```python
from build123d import *

# Parameters (mm, degrees)
BOSS_EXTRUDE1_DEPTH = 44
SHELL1_T            = -2
CUT_EXTRUDE1_DEPTH  = 1


with BuildPart() as part:
    # Sketch1 → Boss-Extrude1 (new body)
    with BuildSketch(Plane(origin=(0, 0, 0), x_dir=(1, 0, 0), z_dir=(0, 1, 0))):
        with BuildLine():
            Line((0, -50), (0, -150))
            ThreePointArc((0, -150), (-86.602540378, -122.474487139), (-141.421356237, -50))
            Line((-141.421356237, -50), (0, -50))
        make_face()
    extrude(amount=BOSS_EXTRUDE1_DEPTH)

    # Shell1
    shell1_openings = [part.faces().sort_by_distance(p)[0] for p in [
        (-56.564232989, 0, 91.421606215),
        (-70.710678119, 22, 50),
        (0, 22, 100),
    ]]
    offset(amount=SHELL1_T, openings=shell1_openings, kind=Kind.INTERSECTION)

    # Sketch3 → Cut-Extrude1 (cut)
    with BuildSketch(Plane.XZ.offset(-42)):
        with BuildLine():
            Line((-139.298241195, 50), (0, 50))
            Line((0, 50), (0, 70))
            Line((0, 70), (-130.399386502, 70))
            ThreePointArc((-130.399386502, 70), (-135.219091094, 60.16475217), (-139.298241195, 50))
        make_face()
    extrude(amount=-CUT_EXTRUDE1_DEPTH, mode=Mode.SUBTRACT)


solid = part.part
```
The model under review builds one solid part; all positions refer to its coordinate system, in mm. A direction names the side the tool comes from. Round coordinates to 2 decimals unless told otherwise and drop trailing zeros. Loops run counter-clockwise (first coordinate to the right, second up) from the corner with the lowest first, then second, coordinate; pieces in that order, holes last. Notation, with made-up numbers: M 73.5,13.25 L 109.5,13.25 A15 ccw 109.5,23.25 Z; hole C 6,37.5 d1. An arc over 180 degrees is marked long. Write item = value, one per line.
Item 1: Take a section at C-C on y = 20. Write out the cut boundary in (x, z), then the cut area to 3 significant figures.
Return value:
outline = M -141.42,50 L -139.3,50 A148 cw 0,148 L 0,150 A150 ccw Z
area = 366 mm2
Item 2: Take a section at B-B on z = 119.5. Write out the cut boundary in (x, y).
Return value:
outline = M -90.66,0 L -87.31,0 L -87.31,42 L 0,42 L 0,44 L -90.66,44 Z
Item 3: Machinability: for faces 1 (the cylindrical face through (-85.54, 21.69, 123.22)), 2 (the flat face through (-71, 43, 60)), which of the approach directions +Z, -Z, +X, -X, +Y, -Y give a long, thin tool a straight path to every point of the face, cutting with its end or side? Answer none if there is none.
Return value:
face_1 = +Z, -X, +Y, -Y
face_2 = -Z, +X, -Y
Item 4: For line 1 (Y direction, x = -28, z = 144.5); line 2 (Y direction, x = -39.5, z = 60.5); line 3 (Z direction, x = -59, y = 15), list the stretches that pass through material, from the lowest coordinate up. Write a range as [from, to].
Return value:
line_1 = [42, 44]
line_2 = [43, 44]
line_3 = [135.73, 137.91]
Item 5: Take a section at A-A on x = -75.5. Write out the cut boundary in (y, z), then the cut area to 3 significant figures.
Return value:
outline = M 0,127.29 L 42,127.29 L 42,70 L 43,70 L 43,50 L 44,50 L 44,129.61 L 0,129.61 Z
area = 237 mm2
Item 6: Take a section at D-D on x = -93. Write out the cut boundary in (y, z).
Return value:
outline = M 0,115.13 L 42,115.13 L 42,70 L 43,70 L 43,50 L 44,50 L 44,117.69 L 0,117.69 Z
Item 7: Insertion check: P1, Ø1, axis at x = -31.5, y = 10, coming from the -Z side; P2, Ø8, axis at x = -63.5, y = 33.5, coming from the +Z side; P3, Ø1.5, axis at x = -28, y = 5.5, coming from the +Z side. Each pin has a flat end and moves straight along its axis. Give the tip position at first contact, or say it passes through.
Return value:
P1 = 144.5
P2 = 137.69
P3 = 147.5
